Read the model definition and answer for the solid it produces. Units are mm, in the model's axes. A direction names the side the tool comes from. Coordinates: 2 decimals unless noted, no trailing zeros. Write each loop counter-clockwise with the first axis right and the second up, starting at its lowest first coordinate (ties: lowest second). Pieces come first, ordered by that corner, then holes. Notation, with made-up numbers: M 22.25,46.5 L 36.25,46.5 A28 ccw 36.25,76.5 Z; hole C -7.5,65 d11. An arc over 180 degrees is marked long. Use a Markdown table: item, result. Add a question column.
Autodesk Inventor part; units mm, degrees
ref_plane "YZ Plane" through (0, 0, 0) normal (1, 0, 0) x (0, 1, 0)
ref_plane "XZ Plane" through (0, 0, 0) normal (0, 1, 0) x (-1, 0, 0)
ref_plane "XY Plane" through (0, 0, 0) normal (0, 0, 1) x (1, 0, 0)
sketch "Sketch1" plane through (0, 0, 0) normal (0, 0, 1) x (1, 0, 0)
  line L0 (0, 0) -> (47.625, 0)
  line L1 (47.625, 0) -> (47.625, 22.5806)
  line L2 (47.625, 22.5806) -> (0, 22.5806)
  line L3 (0, 22.5806) -> (0, 0)
  line L4 (23.8125, 22.5806) -> (23.8125, 9.8806)
  line L5 (23.8125, 9.8806) -> (36.5125, 9.8806)
  line L6 (23.8125, 9.8806) -> (11.1125, 9.8806)
  circle A0 centre (11.1125, 9.8806) radius 3.5687
  circle A1 centre (36.5125, 9.8806) radius 3.5687
  dimension "d1" = 47.625
  dimension "d3" = 12.7
  dimension "d4" = 12.7
  dimension "d5" = 12.7
  dimension "d6" = 7.1374
  dimension "d7" = 7.1374
  dimension "d10" = 22.5806
extrude "Extrusion1" add sketch "Sketch1" along normal blind 6.35
sketch "Sketch3" plane through (0, 0, 6.35) normal (0, 0, 1) x (1, 0, 0)
  line L0 (0, 0) -> (47.625, 0)
  line L1 (23.8125, 0) -> (65.7225, 0)
  line L2 (23.8125, 0) -> (23.8125, -41.91)
  circle A0 centre (23.8125, -41.91) radius 33.02
  line L3 (65.7225, 0) -> (-18.0975, 0)
  line L4 (-18.0975, 0) -> (-18.0975, -83.82)
  line L5 (-18.0975, -83.82) -> (65.7225, -83.82)
  line L6 (65.7225, -83.82) -> (65.7225, 0)
  circle A1 centre (11.1125, 9.8806) radius 3.5687
  line L7 (23.8125, 9.8806) -> (23.8125, -91.7194)
  line L8 (23.8125, 9.8806) -> (125.4125, 9.8806) construction
  line L9 (11.1125, 9.8806) -> (23.8125, 9.8806)
  circle A2 centre (23.8125, -91.7194) radius 3.5687
  line L10 (12.7, -98.0694) -> (34.925, -98.0694)
  line L11 (34.925, -98.0694) -> (34.925, -85.3694)
  line L12 (34.925, -85.3694) -> (12.7, -85.3694)
  line L13 (12.7, -85.3694) -> (12.7, -98.0694)
  line L14 (12.7, -98.0694) -> (34.925, -85.3694) construction
  line L15 (34.925, -98.0694) -> (12.7, -85.3694) construction
  point P0 (12.7, -83.82)
  point P1 (34.925, -83.82)
  dimension "d11" = 41.91
  dimension "d12" = 41.91
  dimension "d13" = 66.04
  dimension "d14" = 83.82
  dimension "d15" = 83.82
  dimension "d19" = 90
  dimension "d20" = 7.1374
  dimension "d22" = 22.225
  dimension "d23" = 12.7
  dimension "d39" = 101.6
extrude "Extrusion2" add sketch "Sketch3" against normal blind 6.35 contours L12 L11 L10 L13 | L0 L2 A0 L7 L5 L4 L3 | L0 L1 L6 L5 L7 A0 L2
sketch "Sketch4" plane through (0, 0, 0) normal (0, 0, -1) x (-1, 0, 0)
  line L0 (-47.625, 22.5806) -> (0, 22.5806)
  line L1 (-23.8125, 22.5806) -> (-23.8125, 0)
  line L2 (-23.8125, 0) -> (-23.8125, -6.8072)
  line L3 (-23.8125, -6.8072) -> (1.143, -6.8072)
  line L4 (-23.8125, -6.8072) -> (-48.7807, -6.8072)
  line L5 (-48.7807, -6.8072) -> (-62.7507, -6.8072)
  line L6 (1.143, -6.8072) -> (15.113, -6.8072)
  line L7 (-62.7507, -6.8072) -> (-62.7507, -20.7772)
  arc A0 (-62.7507, -20.7772) -> (-48.7807, -6.8072) centre (-62.7507, -6.8072) ccw
  line L8 (-62.7507, -20.7772) -> (-62.7507, -45.3517)
  line L9 (-62.7507, -45.3517) -> (8.128, -45.3517)
  line L10 (15.113, -6.8072) -> (15.113, -20.7772)
  arc A1 (1.143, -6.8072) -> (15.113, -20.7772) centre (15.113, -6.8072) ccw
  line L11 (15.113, -20.7772) -> (15.113, -45.3644)
  line L12 (-23.8125, -83.8962) -> (1.143, -83.8962)
  line L13 (-23.8125, -83.8962) -> (-48.7807, -83.8962)
  arc A2 (-48.7807, -83.8962) -> (-62.7507, -69.9262) centre (-62.7507, -83.8962) ccw
  line L14 (-62.7507, -69.9262) -> (-62.7507, -45.3517)
  arc A3 (15.113, -69.9262) -> (1.143, -83.8962) centre (15.113, -83.8962) ccw
  line L15 (15.113, -69.9262) -> (15.113, -45.339)
  point P0 (0, 0)
  dimension "d26" = 6.8072
  dimension "d27" = 24.9555
  dimension "d28" = 24.9682
  dimension "d29" = 13.97
  dimension "d30" = 13.97
  dimension "d31" = 13.97
  dimension "d32" = 13.97
  dimension "d33" = 24.5745
  dimension "d34" = 13.97
  dimension "d35" = 13.97
  dimension "d36" = 24.5872
extrude "Extrusion3" cut sketch "Sketch4" against normal blind 6.35 contours L3 A1 L11 L15 A3 L12 L13 A2 L14 L8 A0 L4
sketch "Sketch5" plane through (0, 0, 6.35) normal (0, 0, 1) x (1, 0, 0)
  line L0 (12.7, -85.3694) -> (34.925, -85.3694)
  line L1 (23.8125, -85.3694) -> (23.8125, -91.7194)
  circle A0 centre (23.8125, -91.7194) radius 3.5687
  point P0 (0, 0)
  dimension "d40" = 6.35
  dimension "d41" = 7.1374
extrude "Extrusion4" cut sketch "Sketch5" against normal blind 7.1374
sketch "Sketch6" plane through (0, 0, 6.35) normal (0, 0, 1) x (1, 0, 0)
  line L0 (-18.0975, -83.82) -> (-1.1432, -83.82)
  line L1 (65.7225, -83.82) -> (48.7809, -83.82)
  line L2 (-1.1432, -83.82) -> (48.7809, -83.82)
  line L3 (12.7, -85.3694) -> (34.925, -85.3694)
  line L4 (34.925, -85.3694) -> (34.925, -83.82)
  line L5 (12.7, -85.3694) -> (12.7, -83.82)
  line L6 (34.925, -85.3694) -> (68.0228, -85.3694)
  line L7 (-18.0975, -85.3694) -> (12.7, -85.3694)
  line L8 (-18.0975, -83.82) -> (-18.0975, -85.3694)
  line L9 (12.7, -98.0694) -> (12.7, -85.3694)
  line L10 (12.7, -85.3694) -> (12.7, -91.7194)
  line L11 (-18.0975, -91.7194) -> (-18.0975, -85.3694)
  line L12 (34.925, -91.7194) -> (68.0228, -91.7194)
  line L13 (65.7225, -83.82) -> (65.7225, -91.7194)
  line L14 (12.7, -91.7194) -> (-12.7, -91.7194)
  line L15 (-12.7, -91.7194) -> (-18.0975, -91.7194)
  line L16 (34.925, -85.3694) -> (34.925, -98.0694)
  line L17 (34.925, -91.7194) -> (34.925, -85.3694)
  point P0 (0, 0)
  point P1 (65.7225, -85.3694)
  dimension "d44" = 6.35
  dimension "d45" = 25.4
extrude "Extrusion5" add sketch "Sketch6" against normal blind 6.35
properties part number "Clamp connector 2"
Item 1: Each of these flat-tipped pins is pushed along its axis until it touches: pin 1 (1.5 mm diameter, centred on y = 8.5, z = 2, fed in from -X); pin 2 (2 mm diameter, centred on x = -6.5, z = 1.5, fed in from +Y); pin 3 (1.9 mm diameter, centred on y = 11.5, z = 3, fed in from +X) (3 decimals). Where does it stop, or does it pass through?
Item 2: Find section B-B on x = 53. Give the vertices of the cut face in (y, z).
Item 3: Find section C-C on x = 22.5. Give the vertices of the cut face in (y, z), then the cut area to 3 significant figures.
Item 4: Find section D-D on z = 1. Give the vertices of the cut face in (x, y) (1 decimal), then the cut area to 3 significant figures.
Item 5: Find section A-A on y = -60.5. Give the vertices of the cut face in (x, z).
Item 6: Determine the mould class of faces 1 (the flat face through (-18.098, -45, 3)), 2 (the flat face through (62.751, -46, 3)), 3 (the flat face through (-15.113, -45, 3)), 4 (the flat face through (57, 0, 3)) for opening direction X: pulls with the +X half, pulls with the -X half, needs draft (parallel to the pull), parting line crosses it, or undercut.
Item 7: Consider probe 1 along Y at (x, z) = (41, 3.5); probe 2 along X at (y, z) = (-29, 1.5); probe 3 along Y at (x, z) = (15, 2.75). Determine where each line is inside the solid, lowest interval first.
Item 8: For faces 5 (the cylindrical face through (-5.371, -73.884, 3.131)), 6 (the flat face through (-9, 0, 3)), 7 (the flat face through (12.7, -95, 3)), 8 (the flat face through (34.925, -95, 3)), determine the directions among +Z, -Z, +X, -X, +Y, -Y from which every point of the face is accessible in a straight line to the end or side of a thin tool.
Geometry says:
| question | item | result |
|---|---|---|
| 1 | pin 1 | stops at x = 0 |
| 1 | pin 2 | stops at y = 0 |
| 1 | pin 3 | stops at x = 47.625 |
| 2 | outline | M -91.72,0 L -73.89,0 L -73.89,6.35 L -91.72,6.35 Z; M -16.81,0 L 0,0 L 0,6.35 L -16.81,6.35 Z |
| 3 | outline | M -98.07,0 L -95.04,0 L -95.04,6.35 L -98.07,6.35 Z; M -88.4,0 L -83.82,0 L -83.82,6.35 L -88.4,6.35 Z; M -6.81,0 L 22.58,0 L 22.58,6.35 L -6.81,6.35 Z |
| 3 | area | 235 mm2 |
| 4 | outline | M -18.1,-91.7 L 12.7,-91.7 L 12.7,-98.1 L 34.9,-98.1 L 34.9,-91.7 L 65.7,-91.7 L 65.7,0 L 47.6,0 L 47.6,22.6 L 0,22.6 L 0,0 L -18.1,0 Z; hole M -15.1,-69.9 A14 cw -1.1,-83.8 L 48.8,-83.8 A14 cw 62.8,-69.9 L 62.8,-20.8 A14 cw 48.8,-6.8 L -1.1,-6.8 A14 cw -15.1,-20.8 Z; hole C 11.1,9.9 d7.1; hole C 23.8,-91.7 d7.1; hole C 36.5,9.9 d7.1 |
| 4 | area | 3,400 mm2 |
| 5 | outline | M -18.1,0 L -15.11,0 L -15.11,6.35 L -18.1,6.35 Z; M 62.75,0 L 65.72,0 L 65.72,6.35 L 62.75,6.35 Z |
| 6 | face 1 | pulls with the -X half |
| 6 | face 2 | undercut |
| 6 | face 3 | undercut |
| 6 | face 4 | needs draft |
| 7 | probe 1 | y = -91.72 to -83.82, -6.81 to 22.58 |
| 7 | probe 2 | x = -18.1 to -15.11, 62.75 to 65.72 |
| 7 | probe 3 | y = -98.07 to -83.82, -6.81 to 22.58 |
| 8 | face 5 | +Z, -Z |
| 8 | face 6 | +Z, -Z, -X, +Y |
| 8 | face 7 | +Z, -Z, -X, -Y |
| 8 | face 8 | +Z, -Z, +X, -Y |
